```python
from build123d import *

# Parameters (mm, degrees)
BASPROSKE_W           = 12
BASPROSKE_H           = 11
TOOTHCUT_DEPTH        = 20.646882704
TEETHCUTS_COUNT       = 20
TEETHCUTS_ANGLE       = 342
BORSKE_R              = 0.4
BORE_DEPTH            = 50.0000508
KES_EKSTR_ZYON1_DEPTH = 20


with BuildPart() as part:
    # BasProSke → Base-Revolve (revolve)
    with BuildSketch(Plane(origin=(0, 0, 0), x_dir=(1, 0, 0), z_dir=(0, 1, 0)), mode=Mode.PRIVATE) as base_revolve_sk:
        with Locations((6, 5.5)):
            Rectangle(BASPROSKE_W, BASPROSKE_H)
    revolve(base_revolve_sk.sketch.rotate(Axis((-10, 0, 0), (1, 0, 0)), 180), axis=Axis((-10, 0, 0), (1, 0, 0)))

    # TooCutSke → ToothCut (cut, through all)
    with BuildSketch(Plane(origin=(0, 0, 0), x_dir=(0, 0, -1), z_dir=(1, 0, 0))):
        with BuildLine():
            ThreePointArc((0.499924007, 8.734705318), (0, 8.749), (-0.499924007, 8.734705318))
            ThreePointArc((-0.499924007, 8.734705318), (-0.824302243, 9.905497836), (-1.485192705, 10.924909509))
            ThreePointArc((-1.485192705, 10.924909509), (0, 11.0254), (1.485192705, 10.924909509))
            ThreePointArc((1.485192705, 10.924909509), (0.824302243, 9.905497836), (0.499924007, 8.734705318))
        make_face()
    toothcut = extrude(amount=TOOTHCUT_DEPTH, mode=Mode.SUBTRACT)

    # TeethCuts: ToothCut ×20 about axis
    teethcuts_axis = Axis((-10, 0, 0), (1, 0, 0))
    for i in range(1, TEETHCUTS_COUNT):
        add(toothcut.rotate(teethcuts_axis, i * TEETHCUTS_ANGLE / (TEETHCUTS_COUNT - 1)), mode=Mode.SUBTRACT)

    # BorSke → Bore (cut, symmetric)
    with BuildSketch(Plane(origin=(0, 0, 0), x_dir=(0, 0, -1), z_dir=(1, 0, 0))):
        with Locations(Location((0, 0, 0), (0, 0, 180))):
            Circle(BORSKE_R)
    extrude(amount=BORE_DEPTH, both=True, mode=Mode.SUBTRACT)

    # Çizim1 → Kes-Ekstrüzyon1 (cut)
    with BuildSketch(Plane(origin=(12, 0, 0), x_dir=(0, 0, -1), z_dir=(1, 0, 0))):
        Polygon((4.214656965, 0), (2.107328483, 3.65), (-2.107328483, 3.65), (-4.214656965, 0), (-2.107328483, -3.65), (2.107328483, -3.65), align=None)
    extrude(amount=-KES_EKSTR_ZYON1_DEPTH, mode=Mode.SUBTRACT)


solid = part.part
```
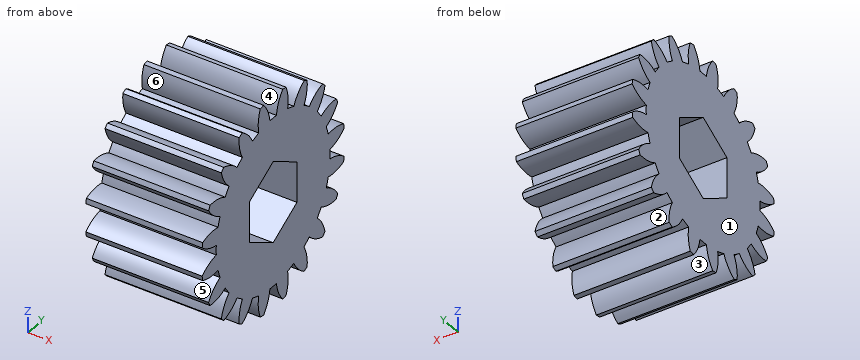
Geometry: final body of the model. Coordinates: model frame, mm. Face numbers are marked on the shaded views. A direction names the side the tool comes from. Give positions to 0.01 mm unless a question says otherwise; leave off trailing zeros. Loops run counter-clockwise (first coordinate to the right, second up) from the corner with the lowest first, then second, coordinate; pieces in that order, holes last. Notation, with made-up numbers: (-14, -6.75) - (10, -6.75) arc R29 ccw to (10, 23.25) - close; hole circle Ø11 at (2, -31.5). An arc over 180 degrees is marked (long way). Answer as CSV lines item,"result". Start each with the question number.
(1) Pin query (flat end, axial travel): P1, Ø4, axis at x = 5, z = 7.5, coming from the -Y side; P2, Ø2, axis at x = 2.5, y = 7.5, coming from the +Z side; P3, Ø1.3, axis at x = 7.5, z = 0.5, coming from the -Y side. Return the tip coordinate at first contact, or that it passes through.
(2) Ray query, line 1 along Y through (x, z) = (11.75, -8.5); line 2 along Y through (x, z) = (6.25, -0.25). Return the intervals inside material, ascending. Write a range as [from, to].
(3) Reachability of the marked faces 4, 5 and 6 from +Z, -Z, +X, -X, +Y, -Y: full face, straight path, thin tool, end or side. Return the list, or none.
(4) Section query A-A (y = -1). Output: boundary loops of the cut face in (x, z), and give its area (3 significant figures).
(5) Mould query, pull axis Z, two halves, no side actions, for the marked faces 1, 2 and 3. Classes: +Z half, -Z half, draft (parallel to the pull), parting line (faces both ways), or undercut.
Worked answers:
1,P1,"stops at y = -7.96"
1,P2,"stops at z = 7.96"
1,P3,"stops at y = -10.49"
2,line 1,"y = [-5.16, -3.36], [-2.23, 2.23], [3.36, 5.16]"
2,line 2,"y = [-8.75, -3.65], [3.65, 8.75]"
3,face 4,"+Z, +X, -X"
3,face 5,"+X, -X, -Y"
3,face 6,"+X, -X"
4,outline,"(0, -10.25) - (12, -10.25) - (12, -3.64) - (0, -3.64) - close; (0, 3.64) - (12, 3.64) - (12, 10.25) - (0, 10.25) - close"
4,area,"159 mm^2"
5,face 1,"draft"
5,face 2,"undercut"
5,face 3,"-Z half"
